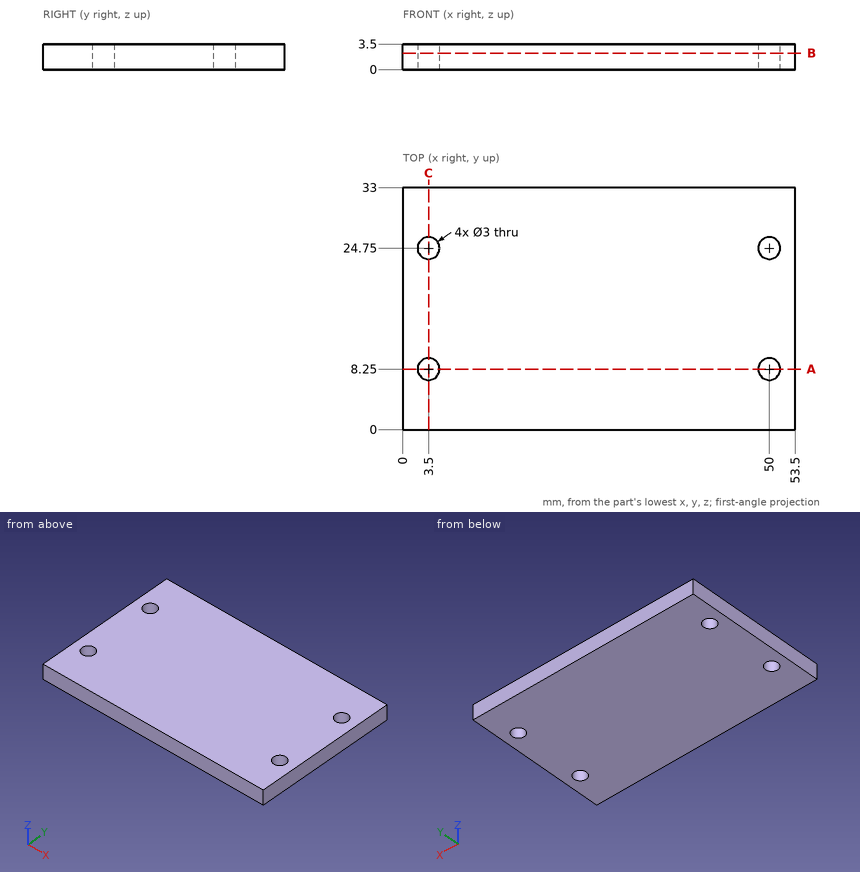
Can you work these out from the drawing? Everything is in mm from the part's minimum corner. Give positions to 0.01 mm unless a question says otherwise; leave off trailing zeros. Loops run counter-clockwise (first coordinate to the right, second up) from the corner with the lowest first, then second, coordinate; pieces in that order, holes last. Notation, with made-up numbers: (43.5, 0) -> (92.5, 0) arc R15 cw to (92.5, 18) -> close; hole circle Ø7 at (10.25, 78). An arc over 180 degrees is marked (long way). Return JSON: item names as keys, results as strings.
Q1. I want a section at B-B, the plane z = 2.25. List the corners of the cut face in (x, y) for me, then the cut area to 3 significant figures.
Checks:
{"outline": "(0, 0) -> (53.5, 0) -> (53.5, 33) -> (0, 33) -> close; hole circle Ø3 at (3.5, 8.25); hole circle Ø3 at (3.5, 24.75); hole circle Ø3 at (50, 8.25); hole circle Ø3 at (50, 24.75)", "area": "1,740 mm2"}
Q2. I need wall thicknesses on probe 1 along Y at (x, z) = (3.5, 1.7); probe 2 along X at (y, z) = (24, 2.25); probe 3 along X at (y, z) = (8, 0.65). Which ranges of each line are inside material? Lowest first, please.
Checks:
{"probe 1": "y = 0 to 6.75, 9.75 to 23.25, 26.25 to 33", "probe 2": "x = 0 to 2.2, 4.8 to 48.7, 51.3 to 53.5", "probe 3": "x = 0 to 2.02, 4.98 to 48.52, 51.48 to 53.5"}
Q3. I want a section at C-C, the plane x = 3.5. List the corners of the cut face in (y, z) for me, then the cut area to 3 significant figures.
Checks:
{"outline": "(0, 0) -> (6.75, 0) -> (6.75, 3.5) -> (0, 3.5) -> close; (9.75, 0) -> (23.25, 0) -> (23.25, 3.5) -> (9.75, 3.5) -> close; (26.25, 0) -> (33, 0) -> (33, 3.5) -> (26.25, 3.5) -> close", "area": "94.5 mm2"}
Q4. I want a section at A-A, the plane y = 8.25. List the corners of the cut face in (x, z) for me, then the cut area to 3 significant figures.
Checks:
{"outline": "(0, 0) -> (2, 0) -> (2, 3.5) -> (0, 3.5) -> close; (5, 0) -> (48.5, 0) -> (48.5, 3.5) -> (5, 3.5) -> close; (51.5, 0) -> (53.5, 0) -> (53.5, 3.5) -> (51.5, 3.5) -> close", "area": "166 mm2"}
Q5. For pin 1 Ø2.5 at (x, y) = (50, 24.75) entering from -Z, with a flat end and sliding along its axis, tell me the tip position at first contact or that it passes through.
Checks:
{"pin 1": "passes through"}
